Autodesk Inventor part; units mm, degrees
ref_plane "YZ Plane" through (0, 0, 0) normal (1, 0, 0) x (0, 1, 0)
ref_plane "XZ Plane" through (0, 0, 0) normal (0, 1, 0) x (-1, 0, 0)
ref_plane "XY Plane" through (0, 0, 0) normal (0, 0, 1) x (1, 0, 0)
sketch "Sketch1" plane through (0, 0, 0) normal (0, 1, 0) x (-1, 0, 0)
  circle A0 centre (0, 0) radius 13
  dimension "d0" = 26
extrude "Extrusion1" add sketch "Sketch1" along normal blind 2
sketch "Sketch2" plane through (0, 2, 0) normal (0, 1, 0) x (1, 0, 0)
  circle A0 centre (0, 0) radius 13 construction
  circle A1 centre (0, 0) radius 10.5
  circle A2 centre (0, 0) radius 6.5
  dimension "d3" = 2.5
  dimension "d4" = 4
extrude "Extrusion2" cut sketch "Sketch2" against normal blind 0.3
sketch "Sketch3" plane through (0, 0, 0) normal (0, -1, 0) x (1, 0, 0)
  circle A0 centre (0, 0) radius 6.25
  dimension "d7" = 12.5
extrude "Extrusion3" cut sketch "Sketch3" against normal blind 0.5
fillet "Fillet1" radius 0.1 5 edges at (13, 2, 0) (-10.5, 2, 0) (-6.5, 2, 0) (13, 0, 0) (-6.25, 0, 0)
properties part number "ThrustWasher" material "Steel, Alloy"
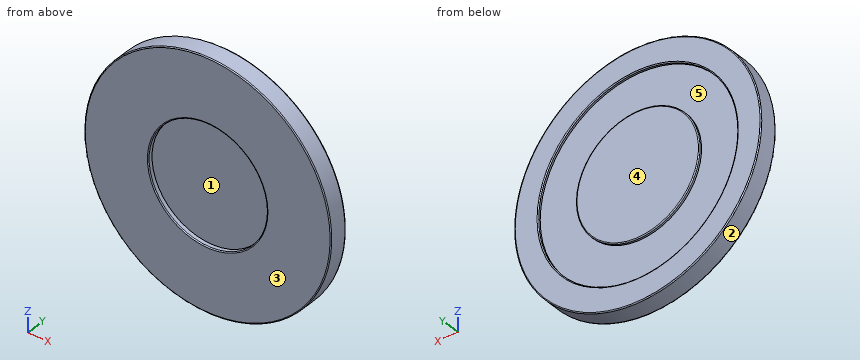
CAD build for the part. Positions are in the model's coordinates, mm. Face numbers are marked on the shaded views. A direction names the side the tool comes from. Round coordinates to 2 decimals unless told otherwise and drop trailing zeros. Loops run counter-clockwise (first coordinate to the right, second up) from the corner with the lowest first, then second, coordinate; pieces in that order, holes last.
(1) Drop flat-ended pins along their axis: pin 1 (2 mm diameter, centred on x = 5, z = 8, fed in from +Y); pin 2 (1 mm diameter, centred on y = 0.5, z = 4.5, fed in from -X). Give the stop position or say it passes through.
(2) Which spindle directions (+Z, -Z, +X, -X, +Y, -Y) get a long thin tool onto all of the face, cutting with end or side? Do the marked faces 4 and 5. Say none if no direction does.
(3) Wall check: line 1 along Z through (x, y) = (0, 0.2); line 2 along X through (y, z) = (1.8, -4.5); line 3 along Y through (x, z) = (-8, -3.75). Give the ranges that are in metal, low to high.
(4) Cut at A-A (x = 0). Give the cut face in (y, z), plus the area to 3 significant figures.
(5) Cut at C-C (y = 0.8). Give the cut face in (x, z), plus the area to 3 significant figures.
(6) Cut at B-B (z = 0). Give the cut face in (x, y).
(7) Two-plate mould, pull along X, no slides. Class the marked faces 1, 2 and 3: +X half, -X half, draft (parallel to the pull), parting line (faces both ways), or undercut.
Findings below:
1. pin 1: stops at y = 1.7
1. pin 2: stops at x = -12.37
2. face 4: +Z, -Z, +X, -X, +Y
2. face 5: +Y
3. line 1: z = -13 to -6.25, 6.25 to 13
3. line 2: x = -12.2 to -9.49, -4.69 to 4.69, 9.49 to 12.2
3. line 3: y = 0 to 1.7
4. outline: (0, -12.9) arc R0.1 ccw to (0.1, -13) - (1.9, -13) arc R0.1 ccw to (2, -12.9) - (2, -10.6) arc R0.1 ccw to (1.9, -10.5) - (1.7, -10.5) - (1.7, -6.5) - (1.9, -6.5) arc R0.1 ccw to (2, -6.4) - (2, 6.4) arc R0.1 ccw to (1.9, 6.5) - (1.7, 6.5) - (1.7, 10.5) - (1.9, 10.5) arc R0.1 ccw to (2, 10.6) - (2, 12.9) arc R0.1 ccw to (1.9, 13) - (0.1, 13) arc R0.1 ccw to (0, 12.9) - (0, 6.35) arc R0.1 ccw to (0.1, 6.25) - (0.5, 6.25) - (0.5, -6.25) - (0.1, -6.25) arc R0.1 ccw to (0, -6.35) - close
4. area: 43.3 mm2
5. outline: circle Ø26 at (0, 0)
5. area: 531 mm2
6. outline: (-13, 0.1) arc R0.1 ccw to (-12.9, 0) - (-6.35, 0) arc R0.1 ccw to (-6.25, 0.1) - (-6.25, 0.5) - (6.25, 0.5) - (6.25, 0.1) arc R0.1 ccw to (6.35, 0) - (12.9, 0) arc R0.1 ccw to (13, 0.1) - (13, 1.9) arc R0.1 ccw to (12.9, 2) - (10.6, 2) arc R0.1 ccw to (10.5, 1.9) - (10.5, 1.7) - (6.5, 1.7) - (6.5, 1.9) arc R0.1 ccw to (6.4, 2) - (-6.4, 2) arc R0.1 ccw to (-6.5, 1.9) - (-6.5, 1.7) - (-10.5, 1.7) - (-10.5, 1.9) arc R0.1 ccw to (-10.6, 2) - (-12.9, 2) arc R0.1 ccw to (-13, 1.9) - close
7. face 1: undercut
7. face 2: parting line
7. face 3: draft
